from build123d import *

# Parameters (mm, degrees)
BOSS_EXTRUDE4_DEPTH = 2.8
SKETCH5_R           = 1.65
SKETCH5_R_2         = 3
CUT_EXTRUDE1_DEPTH  = 3.8


with BuildPart() as part:
    # Sketch2 → Boss-Extrude4 (new body)
    with BuildSketch(Plane(origin=(0, 0, 0), x_dir=(1, 0, 0), z_dir=(0, 1, 0))):
        with BuildLine():
            Line((46, -130), (-46, -130))
            ThreePointArc((-46, -130), (-74.550970119, -119.478980051), (-89.448061775, -92.947368421))
            ThreePointArc((-89.448061775, -92.947368421), (-88.08864154, -88.106685893), (-83.523326079, -86))
            Line((-83.523326079, -86), (-74, -86))
            Line((-74, -86), (-74, -16))
            Line((-74, -16), (-84, -16))
            ThreePointArc((-84, -16), (-88.242640687, -14.242640687), (-90, -10))
            Line((-90, -10), (-90, 10))
            ThreePointArc((-90, 10), (-88.242640687, 14.242640687), (-84, 16))
            Line((-84, 16), (-74, 16))
            Line((-74, 16), (-74, 86))
            Line((-74, 86), (-83.523326079, 86))
            ThreePointArc((-83.523326079, 86), (-88.08864154, 88.106685893), (-89.448061775, 92.947368421))
            ThreePointArc((-89.448061775, 92.947368421), (-74.550970119, 119.478980051), (-46, 130))
            Line((-46, 130), (46, 130))
            ThreePointArc((46, 130), (74.550970119, 119.478980051), (89.448061775, 92.947368421))
            ThreePointArc((89.448061775, 92.947368421), (88.08864154, 88.106685893), (83.523326079, 86))
            Line((83.523326079, 86), (74, 86))
            Line((74, 86), (74, 16))
            Line((74, 16), (84, 16))
            ThreePointArc((84, 16), (88.242640687, 14.242640687), (90, 10))
            Line((90, 10), (90, -10))
            ThreePointArc((90, -10), (88.242640687, -14.242640687), (84, -16))
            Line((84, -16), (74, -16))
            Line((74, -16), (74, -86))
            Line((74, -86), (83.523326079, -86))
            ThreePointArc((83.523326079, -86), (88.08864154, -88.106685893), (89.448061775, -92.947368421))
            ThreePointArc((89.448061775, -92.947368421), (74.550970119, -119.478980051), (46, -130))
        make_face()
    extrude(amount=BOSS_EXTRUDE4_DEPTH)

    # Sketch5 → Cut-Extrude1 (cut, through all)
    with BuildSketch(Plane(origin=(0, 2.8, 0), x_dir=(1, 0, 0), z_dir=(0, 1, 0))):
        with Locations((-69.6, -51)):
            Circle(SKETCH5_R)
        with Locations((-63.25, -51)):
            Circle(SKETCH5_R)
        with Locations((-56.9, -51)):
            Circle(SKETCH5_R)
        with Locations((-50.55, -51)):
            Circle(SKETCH5_R)
        with Locations((-44.2, -51)):
            Circle(SKETCH5_R)
        with Locations((-37.85, -51)):
            Circle(SKETCH5_R)
        with Locations((-31.5, -51)):
            Circle(SKETCH5_R)
        with Locations((31.5, -51)):
            Circle(SKETCH5_R)
        with Locations((37.85, -51)):
            Circle(SKETCH5_R)
        with Locations((44.2, -51)):
            Circle(SKETCH5_R)
        with Locations((50.55, -51)):
            Circle(SKETCH5_R)
        with Locations((56.9, -51)):
            Circle(SKETCH5_R)
        with Locations((63.25, -51)):
            Circle(SKETCH5_R)
        with Locations((69.6, -51)):
            Circle(SKETCH5_R)
        with Locations((69.6, 51)):
            Circle(SKETCH5_R)
        with Locations((63.25, 51)):
            Circle(SKETCH5_R)
        with Locations((56.9, 51)):
            Circle(SKETCH5_R)
        with Locations((50.55, 51)):
            Circle(SKETCH5_R)
        with Locations((44.2, 51)):
            Circle(SKETCH5_R)
        with Locations((37.85, 51)):
            Circle(SKETCH5_R)
        with Locations((31.5, 51)):
            Circle(SKETCH5_R)
        with Locations((-31.5, 51)):
            Circle(SKETCH5_R)
        with Locations((-37.85, 51)):
            Circle(SKETCH5_R)
        with Locations((-44.2, 51)):
            Circle(SKETCH5_R)
        with Locations((-50.55, 51)):
            Circle(SKETCH5_R)
        with Locations((-56.9, 51)):
            Circle(SKETCH5_R)
        with Locations((-63.25, 51)):
            Circle(SKETCH5_R)
        with Locations((-69.6, 51)):
            Circle(SKETCH5_R)
        with Locations((-14, -51)):
            Circle(SKETCH5_R_2)
        with Locations((14, -51)):
            Circle(SKETCH5_R_2)
        with Locations((14, 51)):
            Circle(SKETCH5_R_2)
        with Locations((-14, 51)):
            Circle(SKETCH5_R_2)
        with Locations((-14, 0)):
            Circle(SKETCH5_R_2)
        with Locations((14, 0)):
            Circle(SKETCH5_R_2)
        with Locations((-80, 96)):
            Circle(SKETCH5_R)
        with Locations((-80, 0)):
            Circle(SKETCH5_R)
        with Locations((80, 0)):
            Circle(SKETCH5_R)
        with Locations((-80, -96)):
            Circle(SKETCH5_R)
        with Locations((80, -96)):
            Circle(SKETCH5_R)
        with Locations((80, 96)):
            Circle(SKETCH5_R)
        with Locations((-15, -114)):
            Circle(SKETCH5_R)
        with Locations((15, -114)):
            Circle(SKETCH5_R)
        with Locations((15, 114)):
            Circle(SKETCH5_R)
        with Locations((-15, 114)):
            Circle(SKETCH5_R)
    extrude(amount=-CUT_EXTRUDE1_DEPTH, mode=Mode.SUBTRACT)


solid = part.part
Geometry: final body of the model. Coordinates: model frame, mm. A direction names the side the tool comes from. Give positions to 0.01 mm unless a question says otherwise; leave off trailing zeros. Write each loop counter-clockwise with the first axis right and the second up, starting at its lowest first coordinate (ties: lowest second). Pieces come first, ordered by that corner, then holes. Notation, with made-up numbers: M 11.25,64.5 L 52.25,64.5 A5 cw 52.25,68.5 Z; hole C -30,77.5 d2. An arc over 180 degrees is marked long. Answer in a Markdown table with one row per item. Add a question column.
(1) Mould query, pull axis Z, two halves, no side actions, for faces 4 (the cylindrical face through (74.881, 1.38, 119.195)), 5 (the cylindrical face through (-14, 1, 48)), 6 (the cylindrical face through (88.04, 1.38, 88.05)), 7 (the flat face through (1, 2.8, -2)). Classes: +Z half, -Z half, draft (parallel to the pull), parting line (faces both ways), or undercut.
(2) First-contact query: pin 1 (0.8 mm diameter, centred on x = 78.5, y = 1, fed in from +Z); pin 2 (1.5 mm diameter, centred on x = 71.5, y = 1.5, fed in from -Z); pin 3 (1.4 mm diameter, centred on x = 81, y = 1.5, fed in from -Z). Flat tips, straight axial feed; report the tip coordinate or a pass-through.
(3) Section A-A on y = 2.05. State how many separate pieces and enclosed holes the cut face has, and give its area (3 significant figures).
(4) Reachability of faces 1 (the cylindrical face through (-88.289, 1.38, -14.196)), 2 (the cylindrical face through (88.289, 1.38, 14.196)), 3 (the cylindrical face through (-17, 1, 0)) from +Z, -Z, +X, -X, +Y, -Y: full face, straight path, thin tool, end or side. Return the list, or none.
(5) Ray query, line 1 (X direction, y = 0.6, z = 0); line 2 (X direction, y = 1.55, z = -96); line 3 (Z direction, x = -56.9, y = 1.3). Return the intervals inside material, ascending.
(6) Section B-B on z = 21. Return loops of the section in (x, y), and give its area (3 significant figures).
Result set:
| question | item | result |
|---|---|---|
| 1 | face 4 | +Z half |
| 1 | face 5 | undercut |
| 1 | face 6 | undercut |
| 1 | face 7 | draft |
| 2 | pin 1 | stops at z = 116.09 |
| 2 | pin 2 | stops at z = -122.38 |
| 2 | pin 3 | stops at z = -113.56 |
| 3 | separate pieces | 1 |
| 3 | enclosed holes | 44 |
| 3 | area | 40,100 mm^2 |
| 4 | face 1 | -X, +Y, -Y |
| 4 | face 2 | +X, +Y, -Y |
| 4 | face 3 | +Y, -Y |
| 5 | line 1 | x = -90 to -81.65, -78.35 to -17, -11 to 11, 17 to 78.35, 81.65 to 90 |
| 5 | line 2 | x = -88.85 to -81.65, -78.35 to 78.35, 81.65 to 88.85 |
| 5 | line 3 | z = -128.63 to -52.65, -49.35 to 49.35, 52.65 to 128.63 |
| 6 | outline | M -74,0 L 74,0 L 74,2.8 L -74,2.8 Z |
| 6 | area | 414 mm^2 |
